```python
from build123d import *

# Parameters (mm, degrees)
SKETCH1_W               = 8
SKETCH1_H               = 8
BOSS_EXTRUDE1_DEPTH     = 3
CUT_EXTRUDE1_DEPTH      = 12.704699911
CUT_EXTRUDE1_DEPTH_BACK = 12.704699911
CUT_EXTRUDE2_DEPTH      = 11
SKETCH4_R               = 1.8
CUT_EXTRUDE3_DEPTH      = 0.8
SKETCH5_W               = 8
SKETCH5_H               = 1
BOSS_EXTRUDE2_DEPTH     = 2
FILLET1_R               = 4
CUT_EXTRUDE4_DEPTH      = 0.4


with BuildPart() as part:
    # Sketch1 → Boss-Extrude1 (new body)
    with BuildSketch(Plane(origin=(0, 0, 0), x_dir=(1, 0, 0), z_dir=(0, 1, 0))):
        with Locations((4, 4)):
            Rectangle(SKETCH1_W, SKETCH1_H)
    extrude(amount=BOSS_EXTRUDE1_DEPTH)

    # Sketch2 → Cut-Extrude1 (cut, two sides: drawn at the far end of the back side and taken through both)
    with BuildSketch(Plane.XY.offset(-CUT_EXTRUDE1_DEPTH_BACK)):
        Polygon((0, 0), (0.6, 3), (0, 3), align=None)
        Polygon((8, 0), (7.4, 3), (8, 3), align=None)
    extrude(amount=CUT_EXTRUDE1_DEPTH + CUT_EXTRUDE1_DEPTH_BACK, mode=Mode.SUBTRACT)

    # Sketch3 → Cut-Extrude2 (cut)
    with BuildSketch(Plane(origin=(0, 0, 0), x_dir=(0, 0, -1), z_dir=(1, 0, 0))):
        Polygon((0, 0), (0.6, 3), (0, 3), align=None)
        Polygon((8, 3), (7.4, 3), (8, 0), align=None)
    extrude(amount=CUT_EXTRUDE2_DEPTH, mode=Mode.SUBTRACT)

    # Sketch4 → Cut-Extrude3 (cut)
    with BuildSketch(Plane.XZ):
        with Locations(Location((4, -3.75, 0), (0, 0, 270))):
            Circle(SKETCH4_R)
    extrude(amount=-CUT_EXTRUDE3_DEPTH, mode=Mode.SUBTRACT)

    # Sketch5 → Boss-Extrude2 (add)
    with BuildSketch(Plane.XZ):
        with Locations((4, -7.5)):
            Rectangle(SKETCH5_W, SKETCH5_H)
    extrude(amount=BOSS_EXTRUDE2_DEPTH)

    # Fillet1
    # the kernel refuses this fillet: 4 mm, written as the material it takes off along each edge
    with BuildSketch(Plane(origin=(8, -2, -16.660254038), x_dir=(0, 1, 0), z_dir=(0, 0, 1)), Plane(origin=(0, -2, 1.660254038), x_dir=(0, 1, 0), z_dir=(0, 0, -1))) as fillet1_piece_1:
        with BuildLine():
            CenterArc((4, 3.464101615), FILLET1_R, 180, 60)
            Line((0, 3.464101615), (-0.08, 3.464101615))
            Line((-0.08, 3.464101615), (-0.08, 0))
            Line((-0.08, 0), (0, -0.08))
            ThreePointArc((0, -0.08), (1, -0.08), (1.96, -0.069282032))
            Line((1.96, -0.069282032), (2, 0))
        make_face()
    extrude(amount=18.320508076, mode=Mode.SUBTRACT)

    # Sketch6 → Cut-Extrude4 (cut)
    with BuildSketch(Plane(origin=(0, 3, 0), x_dir=(1, 0, 0), z_dir=(0, 1, 0))):
        Polygon((2.312898911, 2.049121591), (2.312898911, 6.049121591), (3.08212968, 6.049121591), (3.08212968, 4.258256206), (4.768828398, 6.049121591), (5.825719424, 6.049121591), (4.306488654, 4.502647232), (5.877001475, 2.049121591), (4.852161731, 2.049121591), (3.723155321, 3.907294667), (3.08212968, 3.255051078), (3.08212968, 2.049121591), align=None)
    extrude(amount=-CUT_EXTRUDE4_DEPTH, mode=Mode.SUBTRACT)


solid = part.part
```
Input: part model. Units: mm. Frame: model coordinates. A direction names the side the tool comes from. Round coordinates to 2 decimals unless told otherwise and drop trailing zeros. Loops run counter-clockwise (first coordinate to the right, second up) from the corner with the lowest first, then second, coordinate; pieces in that order, holes last. Notation, with made-up numbers: (38, 3.25) -> (84, 3.25) arc R23 ccw to (84, 12.25) -> close; hole circle Ø1 at (-31.5, 27). An arc over 180 degrees is marked (long way). Write each question's results on one line, items separated by ' | '.
1. Section D-D (y = 1.35). Return loops of the section in (x, z).
Geometry results:
outline: (0.27, -7.73) -> (7.73, -7.73) -> (7.73, -0.27) -> (0.27, -0.27) -> close
2. Section A-A (y = 0.45). Return loops of the section in (x, z), and give its area (3 significant figures).
Geometry results:
outline: (0.09, -7.91) -> (7.91, -7.91) -> (7.91, -0.09) -> (0.09, -0.09) -> close; hole circle Ø3.6 at (4, -3.75) | area: 51.0 mm2
3. Ray query, line 1 (Z direction, x = 4, y = -1.3); line 2 (Y direction, x = 5, z = -4.25); line 3 (Y direction, x = 4.75, z = -0.75). Return the intervals inside material, ascending. Write a range as from..to.
Geometry results:
line 1: -8..-7 | line 2: 0.8..3 | line 3: 0..3
4. First-contact query: P1, Ø3, axis at x = 1.5, z = -3, coming from the -Y side; P2, Ø3, axis at x = 4, z = -3.5, coming from the +Y side; P3, Ø1.5, axis at x = 2, y = -1.5, coming from the +Z side; P4, Ø2, axis at x = 3.5, z = -3.5, coming from the -Y side. Flat tips, straight axial feed; report the tip coordinate or a pass-through.
Geometry results:
P1: y = 0 | P2: y = 3 | P3: z = -7 | P4: y = 0.8
5. Section C-C (z = -5). Return loops of the section in (x, y), and give its area (3 significant figures).
Geometry results:
outline: (0, 0) -> (2.7, 0) -> (2.7, 0.8) -> (5.3, 0.8) -> (5.3, 0) -> (8, 0) -> (7.4, 3) -> (4.8, 3) -> (4.8, 2.6) -> (3.78, 2.6) -> (3.78, 3) -> (3.08, 3) -> (3.08, 2.6) -> (2.31, 2.6) -> (2.31, 3) -> (0.6, 3) -> close | area: 19.4 mm2
6. Section B-B (x = 6.25). Return loops of the section in (y, z), and give its area (3 significant figures).
Geometry results:
outline: (-1.61, -8) -> (0, -8) -> (3, -7.4) -> (3, -0.6) -> (0, 0) -> (0, -7) -> (-1.61, -7) -> close | area: 23.8 mm2
7. Set-up query: faces 1 (the face through (4.541, 0.394, -5.467)), 2 (the face through (5.08, 2.8, -5.29)), 3 (the face through (4, -1, -7)), 4 (the face through (6.51, -1.48, -7.51)). Return all of +Z, -Z, +X, -X, +Y, -Y with unobstructed straight access to the full face (end or side cutting, diameter ignored); none if empty.
Geometry results:
face 1: -Y | face 2: +Y | face 3: +Z, +X, -X, -Y | face 4: +Z, -Z, +X, -Y
8. Mould query, pull axis Z, two halves, no side actions, for faces 5 (the face through (3.9, 1.5, -7.7)), 6 (the face through (3, 0, -2)), 7 (the face through (5.081, 2.803, -3.293)). Classes: +Z half, -Z half, draft (parallel to the pull), parting line (faces both ways), or undercut.
Geometry results:
face 5: -Z half | face 6: draft | face 7: undercut
